from build123d import *

# Parameters (mm, degrees)
SKETCH1_R           = 1.5
BOSS_EXTRUDE1_DEPTH = 3
SKETCH2_R           = 1.5
SKETCH2_R_2         = 2
SKETCH2_W           = 9
SKETCH2_H           = 13.2
CUT_EXTRUDE1_DEPTH  = 4
SKETCH3_R           = 1.5
CUT_EXTRUDE2_DEPTH  = 4


with BuildPart() as part:
    # Sketch1 → Boss-Extrude1 (new body)
    with BuildSketch(Plane(origin=(0, 0, 0), x_dir=(1, 0, 0), z_dir=(0, 1, 0))):
        with BuildLine():
            Line((-72, 110), (-48, 110))
            ThreePointArc((-48, 110), (-45.878679656, 109.121320344), (-45, 107))
            Line((-45, 107), (-45, 100))
            Line((-45, 100), (-74.819077862, 18.072756904))
            ThreePointArc((-74.819077862, 18.072756904), (-74.954423259, 17.567641007), (-75, 17.046696474))
            Line((-75, 17.046696474), (-75, -127))
            ThreePointArc((-75, -127), (-74.121320344, -129.121320344), (-72, -130))
            Line((-72, -130), (72, -130))
            ThreePointArc((72, -130), (74.121320344, -129.121320344), (75, -127))
            Line((75, -127), (75, 17.046696474))
            ThreePointArc((75, 17.046696474), (74.954423259, 17.567641007), (74.819077862, 18.072756904))
            Line((74.819077862, 18.072756904), (45, 100))
            Line((45, 100), (45, 107))
            ThreePointArc((45, 107), (45.878679656, 109.121320344), (48, 110))
            Line((48, 110), (72, 110))
            ThreePointArc((72, 110), (74.121320344, 110.878679656), (75, 113))
            Line((75, 113), (75, 127))
            ThreePointArc((75, 127), (74.121320344, 129.121320344), (72, 130))
            Line((72, 130), (-72, 130))
            ThreePointArc((-72, 130), (-74.121320344, 129.121320344), (-75, 127))
            Line((-75, 127), (-75, 113))
            ThreePointArc((-75, 113), (-74.121320344, 110.878679656), (-72, 110))
        make_face()
        with Locations((-71, -126)):
            Circle(SKETCH1_R, mode=Mode.SUBTRACT)
        with Locations((-71, 16.870369494)):
            Circle(SKETCH1_R, mode=Mode.SUBTRACT)
        with Locations((71, -126)):
            Circle(SKETCH1_R, mode=Mode.SUBTRACT)
        with Locations((71, 16.870369494)):
            Circle(SKETCH1_R, mode=Mode.SUBTRACT)
        with Locations((-71, 126)):
            Circle(SKETCH1_R, mode=Mode.SUBTRACT)
        with Locations((-71, 114)):
            Circle(SKETCH1_R, mode=Mode.SUBTRACT)
        with Locations((71, 114)):
            Circle(SKETCH1_R, mode=Mode.SUBTRACT)
        with Locations((71, 126)):
            Circle(SKETCH1_R, mode=Mode.SUBTRACT)
        with BuildLine():
            Line((19, 102.5), (-19, 102.5))
            ThreePointArc((-19, 102.5), (-19.707106781, 102.792893219), (-20, 103.5))
            Line((-20, 103.5), (-20, 106.5))
            ThreePointArc((-20, 106.5), (-19.707106781, 107.207106781), (-19, 107.5))
            Line((-19, 107.5), (19, 107.5))
            ThreePointArc((19, 107.5), (19.707106781, 107.207106781), (20, 106.5))
            Line((20, 106.5), (20, 103.5))
            ThreePointArc((20, 103.5), (19.707106781, 102.792893219), (19, 102.5))
        make_face(mode=Mode.SUBTRACT)
    extrude(amount=BOSS_EXTRUDE1_DEPTH)

    # Sketch2 → Cut-Extrude1 (cut)
    with BuildSketch(Plane(origin=(0, 3, 0), x_dir=(1, 0, 0), z_dir=(0, 1, 0))):
        with Locations((-46.875, -60.1)):
            Circle(SKETCH2_R)
        with Locations((-63.125, -29.9)):
            Circle(SKETCH2_R)
        with Locations((-63.125, -60.1)):
            Circle(SKETCH2_R)
        with Locations((-46.875, -29.9)):
            Circle(SKETCH2_R)
        with Locations((22, 27)):
            Circle(SKETCH2_R)
        with Locations((22, -17)):
            Circle(SKETCH2_R)
        with Locations((-22, -17)):
            Circle(SKETCH2_R)
        with Locations((-22, 27)):
            Circle(SKETCH2_R)
        with Locations((65, -115)):
            Circle(SKETCH2_R)
        with Locations((-65, -115)):
            Circle(SKETCH2_R)
        with Locations((3.75, 92.5)):
            Circle(SKETCH2_R_2)
        with Locations((63.125, -60.1)):
            Circle(SKETCH2_R)
        with Locations((46.875, -60.1)):
            Circle(SKETCH2_R)
        with Locations((65.875, -20.1)):
            Circle(SKETCH2_R)
        with BuildLine():
            Line((64, -11.5), (46, -11.5))
            ThreePointArc((46, -11.5), (45.292893219, -11.207106781), (45, -10.5))
            Line((45, -10.5), (45, -7.5))
            ThreePointArc((45, -7.5), (45.292893219, -6.792893219), (46, -6.5))
            Line((46, -6.5), (64, -6.5))
            ThreePointArc((64, -6.5), (64.707106781, -6.792893219), (65, -7.5))
            Line((65, -7.5), (65, -10.5))
            ThreePointArc((65, -10.5), (64.707106781, -11.207106781), (64, -11.5))
        make_face()
        with Locations((55, 5)):
            Rectangle(SKETCH2_W, SKETCH2_H)
        with BuildLine():
            Line((-64, -15.5), (-46, -15.5))
            ThreePointArc((-46, -15.5), (-45.292893219, -15.792893219), (-45, -16.5))
            Line((-45, -16.5), (-45, -19.5))
            ThreePointArc((-45, -19.5), (-45.292893219, -20.207106781), (-46, -20.5))
            Line((-46, -20.5), (-64, -20.5))
            ThreePointArc((-64, -20.5), (-64.707106781, -20.207106781), (-65, -19.5))
            Line((-65, -19.5), (-65, -16.5))
            ThreePointArc((-65, -16.5), (-64.707106781, -15.792893219), (-64, -15.5))
        make_face()
        with BuildLine():
            Line((-45, -73.5), (-45, -70.5))
            ThreePointArc((-45, -70.5), (-45.292893219, -69.792893219), (-46, -69.5))
            Line((-46, -69.5), (-64, -69.5))
            ThreePointArc((-64, -69.5), (-64.707106781, -69.792893219), (-65, -70.5))
            Line((-65, -70.5), (-65, -73.5))
            ThreePointArc((-65, -73.5), (-64.707106781, -74.207106781), (-64, -74.5))
            Line((-64, -74.5), (-46, -74.5))
            ThreePointArc((-46, -74.5), (-45.292893219, -74.207106781), (-45, -73.5))
        make_face()
        with BuildLine():
            Line((38, -50), (36, -50))
            ThreePointArc((36, -50), (35.292893219, -50.292893219), (35, -51))
            Line((35, -51), (35, -119))
            ThreePointArc((35, -119), (35.292893219, -119.707106781), (36, -120))
            Line((36, -120), (38, -120))
            ThreePointArc((38, -120), (38.707106781, -119.707106781), (39, -119))
            Line((39, -119), (39, -51))
            ThreePointArc((39, -51), (38.707106781, -50.292893219), (38, -50))
        make_face()
        with BuildLine():
            Line((-35, -51), (-35, -119))
            ThreePointArc((-35, -119), (-35.292893219, -119.707106781), (-36, -120))
            Line((-36, -120), (-38, -120))
            ThreePointArc((-38, -120), (-38.707106781, -119.707106781), (-39, -119))
            Line((-39, -119), (-39, -51))
            ThreePointArc((-39, -51), (-38.707106781, -50.292893219), (-38, -50))
            Line((-38, -50), (-36, -50))
            ThreePointArc((-36, -50), (-35.292893219, -50.292893219), (-35, -51))
        make_face()
        with BuildLine():
            Line((-5.5, 94.5), (-1.5, 94.5))
            ThreePointArc((-1.5, 94.5), (0.5, 92.5), (-1.5, 90.5))
            Line((-1.5, 90.5), (-5.5, 90.5))
            ThreePointArc((-5.5, 90.5), (-7.5, 92.5), (-5.5, 94.5))
        make_face()
        with BuildLine():
            Line((-14, 60), (14, 60))
            ThreePointArc((14, 60), (14.707106781, 59.707106781), (15, 59))
            Line((15, 59), (15, 56))
            ThreePointArc((15, 56), (14.707106781, 55.292893219), (14, 55))
            Line((14, 55), (-14, 55))
            ThreePointArc((-14, 55), (-14.707106781, 55.292893219), (-15, 56))
            Line((-15, 56), (-15, 59))
            ThreePointArc((-15, 59), (-14.707106781, 59.707106781), (-14, 60))
        make_face()
        with BuildLine():
            Line((29.5, -10), (26.5, -10))
            ThreePointArc((26.5, -10), (25.792893219, -9.707106781), (25.5, -9))
            Line((25.5, -9), (25.5, 19))
            ThreePointArc((25.5, 19), (25.792893219, 19.707106781), (26.5, 20))
            Line((26.5, 20), (29.5, 20))
            ThreePointArc((29.5, 20), (30.207106781, 19.707106781), (30.5, 19))
            Line((30.5, 19), (30.5, -9))
            ThreePointArc((30.5, -9), (30.207106781, -9.707106781), (29.5, -10))
        make_face()
        with BuildLine():
            Line((-29.5, 20), (-26.5, 20))
            ThreePointArc((-26.5, 20), (-25.792893219, 19.707106781), (-25.5, 19))
            Line((-25.5, 19), (-25.5, -9))
            ThreePointArc((-25.5, -9), (-25.792893219, -9.707106781), (-26.5, -10))
            Line((-26.5, -10), (-29.5, -10))
            ThreePointArc((-29.5, -10), (-30.207106781, -9.707106781), (-30.5, -9))
            Line((-30.5, -9), (-30.5, 19))
            ThreePointArc((-30.5, 19), (-30.207106781, 19.707106781), (-29.5, 20))
        make_face()
        with BuildLine():
            Line((64, -74.5), (46, -74.5))
            ThreePointArc((46, -74.5), (45.292893219, -74.207106781), (45, -73.5))
            Line((45, -73.5), (45, -70.5))
            ThreePointArc((45, -70.5), (45.292893219, -69.792893219), (46, -69.5))
            Line((46, -69.5), (64, -69.5))
            ThreePointArc((64, -69.5), (64.707106781, -69.792893219), (65, -70.5))
            Line((65, -70.5), (65, -73.5))
            ThreePointArc((65, -73.5), (64.707106781, -74.207106781), (64, -74.5))
        make_face()
    extrude(amount=-CUT_EXTRUDE1_DEPTH, mode=Mode.SUBTRACT)

    # Sketch3 → Cut-Extrude2 (cut)
    with BuildSketch(Plane(origin=(0, 3, 0), x_dir=(1, 0, 0), z_dir=(0, 1, 0))):
        with Locations((23.1, 30.81)):
            Circle(SKETCH3_R)
        with Locations((-28.8, 26.11)):
            Circle(SKETCH3_R)
        with Locations((22, -17)):
            Circle(SKETCH3_R)
        with Locations((-40, 70)):
            Circle(SKETCH3_R)
        with Locations((40, 70)):
            Circle(SKETCH3_R)
        with BuildLine():
            Line((-19, -21), (19, -21))
            ThreePointArc((19, -21), (19.707106781, -21.292893219), (20, -22))
            Line((20, -22), (20, -24))
            ThreePointArc((20, -24), (19.707106781, -24.707106781), (19, -25))
            Line((19, -25), (-19, -25))
            ThreePointArc((-19, -25), (-19.707106781, -24.707106781), (-20, -24))
            Line((-20, -24), (-20, -22))
            ThreePointArc((-20, -22), (-19.707106781, -21.292893219), (-19, -21))
        make_face()
    extrude(amount=-CUT_EXTRUDE2_DEPTH, mode=Mode.SUBTRACT)


solid = part.part
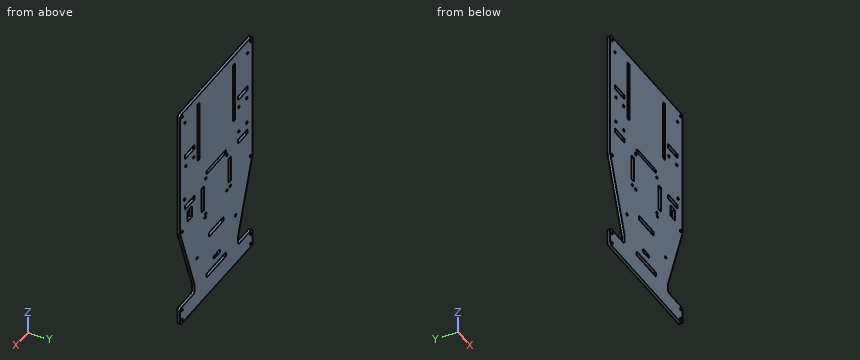
Design review of the part built by this model. Coordinates are the model's own, in mm. Coordinates: 2 decimals unless noted, no trailing zeros. Order: outer loops, then holes, each group sorted by start corner. A loop starts at its lowest first (then second) coordinate and runs counter-clockwise, first axis right, second up. Notation, with made-up numbers: (-34.5, -20.75) -> (6.5, -20.75) arc R18 ccw to (6.5, 2.25) -> close; hole circle Ø4 at (38.25, -30.5). An arc over 180 degrees is marked (long way). One line per item, written item: value.
1) To check wall thickness, follow probe 1 along X at (y, z) = (0.7, 107); probe 2 along X at (y, z) = (2.15, 115); probe 3 along X at (y, z) = (1, 17). State the ranges of each line that lie inside material, in increasing order. Write a range as [from, to].
Output values:
probe 1: x = [-75, -39], [-35, 35], [39, 75]
probe 2: x = [-75, -66.5], [-63.5, -39], [-35, 35], [39, 63.5], [66.5, 75]
probe 3: x = [-75, -65], [-45, -23.5], [-20.5, 20.5], [23.5, 75]
2) Clearance check with flat-ended pins moving along their axes: P1, Ø4, axis at x = 57, z = -5, coming from the -Y side; P2, Ø1.5, axis at y = 1.5, z = -104, coming from the -X side. State where each tip first meets the part, or that it passes through.
Output values:
P1: passes through
P2: stops at x = -45
3) We need section C-C, the plane y = 1.2. Count the separate pieces of the cut face and the enclosed holes in it, then the cut area to 3 significant figures.
Output values:
separate pieces: 1
enclosed holes: 39
area: 33,800 mm2
4) We need section B-B, the plane x = -52.5. Give the boundary of the cut face in (y, z).
Output values:
outline: (0, -130) -> (3, -130) -> (3, -110) -> (0, -110) -> close; (0, -79.39) -> (3, -79.39) -> (3, 15.5) -> (0, 15.5) -> close; (0, 20.5) -> (3, 20.5) -> (3, 69.5) -> (0, 69.5) -> close; (0, 74.5) -> (3, 74.5) -> (3, 130) -> (0, 130) -> close
5) We need section A-A, the plane z = -4.5. Give the boundary of the cut face in (x, y), then the cut area to 3 significant figures.
Output values:
outline: (-75, 0) -> (-30.5, 0) -> (-30.5, 3) -> (-75, 3) -> close; (-25.5, 0) -> (25.5, 0) -> (25.5, 3) -> (-25.5, 3) -> close; (30.5, 0) -> (50.5, 0) -> (50.5, 3) -> (30.5, 3) -> close; (59.5, 0) -> (75, 0) -> (75, 3) -> (59.5, 3) -> close
area: 393 mm2
